```python
from build123d import *

# Parameters (mm, degrees)
BOX_W     = 300
BOX_H     = 300
BOX_DEPTH = 300


with BuildPart() as part:
    # Sketch → Revolution (revolve)
    with BuildSketch(Plane.XZ):
        with BuildLine():
            Line((0, 36), (0, 34))
            Line((0, 34), (17.1, 34))
            add(Edge.make_bspline(
                [(44.08, 0), (44.08, 29.242706), (17.1, 34)],
                knots=[1.570796, 1.570796, 1.570796, 2.978183, 2.978183, 2.978183], degree=2, weights=[1, 0.762458, 1]))
            Line((44.08, 0), (46.08, 0))
            add(Edge.make_bspline(
                [(46.08, 0), (46.08, 35.999994), (17.1, 36)],
                knots=[4.712389, 4.712389, 4.712389, 6.283185, 6.283185, 6.283185], degree=2, weights=[1, 0.707107, 1]))
            Line((17.1, 36), (0, 36))
        make_face()
    revolve(axis=Axis((0, 0, 0), (0, 0, 1)))

    # Box → Box (cut)
    with BuildSketch(Plane(origin=(-86, -8, 0), x_dir=(1, 0, 0), z_dir=(0, -1, 0))):
        with Locations((150, 150)):
            Rectangle(BOX_W, BOX_H)
    box = extrude(amount=BOX_DEPTH, mode=Mode.SUBTRACT)

    # Mirrored: Box across XZ
    add(box.mirror(Plane.XZ), mode=Mode.SUBTRACT)


solid = part.part
```
Can you work these out from the model? Positions are in its coordinate system, mm. Coordinates: 2 decimals unless noted, no trailing zeros. Write each loop counter-clockwise with the first axis right and the second up, starting at its lowest first coordinate (ties: lowest second). Pieces come first, ordered by that corner, then holes. Notation, with made-up numbers: (57, 3.25) - (111, 3.25) arc R20 ccw to (111, 8.25) - close; hole circle Ø10 at (13, 79.5). An arc over 180 degrees is marked (long way). Return JSON: item names as keys, results as strings.
Q1. I'm going to push flat-ended pins straight in: pin 1 Ø1.5 at (x, y) = (-29, 4.5) entering from +Z; pin 2 Ø3 at (y, z) = (2, 11.5) entering from +X; pin 3 Ø5 at (y, z) = (-5.5, 25) entering from -X. Where does each tip first touch, or does it pass through?
Computed values:
{"pin 1": "stops at z = 33.05", "pin 2": "stops at x = 44.9", "pin 3": "stops at x = -39.37"}
Q2. Thinking about a two-plate mould opening in X: for faces 1 (the flat face through (0, 0, 34)), 2 (the flat face through (45, 0, 0)), which applies, +X half, -X half, draft (parallel to the pull), parting line (faces both ways), or undercut?
Computed values:
{"face 1": "undercut", "face 2": "draft"}
Q3. If we section it at A-A (x = -1.5): Please give me the cut outline in (y, z).
Computed values:
{"outline": "(-8, 34) - (8, 34) - (8, 36) - (-8, 36) - close"}
Q4. Please list where these lines run through material, in increasing order: L1, parallel to X at y = 1.5, z = 9.5; L2, parallel to X at y = -6, z = 22.5; L3, parallel to Z at x = -9.5, y = 5.5. Write a range as from..to.
Computed values:
{"L1": "x = -45.03..-42.81, 42.81..45.03", "L2": "x = -39.27..-35.76, 35.76..39.27", "L3": "z = 34..36"}
